```python
from build123d import *

# Parameters (mm, degrees)
ESQUISSE1_W                  = 760
ESQUISSE1_H                  = 40
BOSS_EXTRU_1_DEPTH           = 10
ENL_V_MAT_EXTRU_1_DEPTH      = 762.117599324
ENL_V_MAT_EXTRU_1_DEPTH_BACK = 762.117599324
ENL_V_MAT_EXTRU_2_DEPTH      = 762.117599324
ENL_V_MAT_EXTRU_2_DEPTH_BACK = 762.117599324
ENL_V_MAT_EXTRU_3_DEPTH      = 762.117599324
ENL_V_MAT_EXTRU_3_DEPTH_BACK = 762.117599324
ESQUISSE4_R                  = 4
CONG_1_R                     = 3
CHANFREIN1_SIZE              = 25
ENL_V_MAT_EXTRU_4_DEPTH      = 762.117599324
ENL_V_MAT_EXTRU_4_DEPTH_BACK = 762.117599324
ESQUISSE5_R                  = 2.25
ESQUISSE5_R_2                = 5
ESQUISSE5_R_3                = 2
CONG_2_R                     = 3
CONG_3_R                     = 10


with BuildPart() as part:
    # Esquisse1 → Boss.-Extru.1 (new body)
    with BuildSketch(Plane.XY):
        with Locations((380, 20)):
            Rectangle(ESQUISSE1_W, ESQUISSE1_H)
    extrude(amount=BOSS_EXTRU_1_DEPTH)

    # Esquisse2 → Enlèv. mat.-Extru.1 (cut, two sides: drawn at the far end of the back side and taken through both)
    with BuildSketch(Plane.XY.offset(10).offset(-ENL_V_MAT_EXTRU_1_DEPTH_BACK)):
        Polygon((0, 40), (60, 40), (0, 20), align=None)
    extrude(amount=ENL_V_MAT_EXTRU_1_DEPTH + ENL_V_MAT_EXTRU_1_DEPTH_BACK, mode=Mode.SUBTRACT)

    # Esquisse3 → Enlèv. mat.-Extru.2 (cut, two sides: drawn at the far end of the back side and taken through both)
    with BuildSketch(Plane.XY.offset(10).offset(-ENL_V_MAT_EXTRU_2_DEPTH_BACK)):
        with BuildLine():
            Line((75, 25), (505, 25))
            ThreePointArc((505, 25), (510, 20), (505, 15))
            Line((505, 15), (75, 15))
            ThreePointArc((75, 15), (70, 20), (75, 25))
        make_face()
    extrude(amount=ENL_V_MAT_EXTRU_2_DEPTH + ENL_V_MAT_EXTRU_2_DEPTH_BACK, mode=Mode.SUBTRACT)

    # Esquisse4 → Enlèv. mat.-Extru.3 (cut, two sides: drawn at the far end of the back side and taken through both)
    with BuildSketch(Plane.XY.offset(10).offset(-ENL_V_MAT_EXTRU_3_DEPTH_BACK)):
        with Locations(Location((530, 10, 0), (0, 0, 180))):
            Circle(ESQUISSE4_R)
        with Locations(Location((550, 30, 0), (0, 0, 180))):
            Circle(ESQUISSE4_R)
    extrude(amount=ENL_V_MAT_EXTRU_3_DEPTH + ENL_V_MAT_EXTRU_3_DEPTH_BACK, mode=Mode.SUBTRACT)

    # Congé1
    cong_1_edges = [part.edges().sort_by_distance(p)[0] for p in [
        (0, 20, 5),
        (0, 0, 5),
    ]]
    fillet(cong_1_edges, radius=CONG_1_R)

    # Chanfrein1
    chanfrein1_edges = [part.edges().sort_by_distance(p)[0] for p in [
        (760, 0, 5),
    ]]
    chamfer(chanfrein1_edges, length=CHANFREIN1_SIZE)

    # Esquisse5 → Enlèv. mat.-Extru.4 (cut, two sides: drawn at the far end of the back side and taken through both)
    with BuildSketch(Plane.XY.offset(10).offset(-ENL_V_MAT_EXTRU_4_DEPTH_BACK)):
        with Locations(Location((710, 20, 0), (0, 0, 180))):
            Circle(ESQUISSE5_R)
        with Locations(Location((668, 20, 0), (0, 0, 180))):
            Circle(ESQUISSE5_R)
        with Locations(Location((630, 30, 0), (0, 0, 180))):
            Circle(ESQUISSE5_R_2)
        with Locations(Location((605, 25, 0), (0, 0, 180))):
            Circle(ESQUISSE5_R_3)
    extrude(amount=ENL_V_MAT_EXTRU_4_DEPTH + ENL_V_MAT_EXTRU_4_DEPTH_BACK, mode=Mode.SUBTRACT)

    # Congé2
    cong_2_edges = [part.edges().sort_by_distance(p)[0] for p in [
        (760, 40, 5),
    ]]
    fillet(cong_2_edges, radius=CONG_2_R)

    # Congé3
    cong_3_edges = [part.edges().sort_by_distance(p)[0] for p in [
        (760, 25, 5),
        (735, 0, 5),
    ]]
    fillet(cong_3_edges, radius=CONG_3_R)


solid = part.part
```
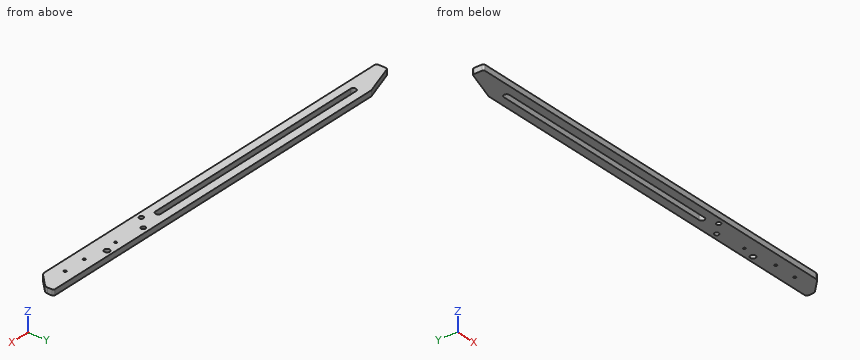
Source: CAD feature listing. Evaluate the final solid. Frame: model axes, mm. Round coordinates to 2 decimals unless told otherwise and drop trailing zeros. Order: outer loops, then holes, each group sorted by start corner. A loop starts at its lowest first (then second) coordinate and runs counter-clockwise, first axis right, second up. Notation, with made-up numbers: (78, 23.25) -> (120, 23.25) arc R23 ccw to (120, 49.25) -> close; hole circle Ø8 at (76, -38.5). An arc over 180 degrees is marked (long way). One line per item, written item: value. Start each with the question number.
Q1. Pin query (flat end, axial travel): pin 1 (1 mm diameter, centred on y = 14.5, z = 8, fed in from +X); pin 2 (5 mm diameter, centred on y = 22.5, z = 7.5, fed in from -X). Return the tip coordinate at first contact, or that it passes through.
Q2. Section query A-A (x = 111). Return the cut outline in (y, z), plus the area to 3 significant figures.
Q3. Section query B-B (z = 2). Return the cut outline in (x, y), plus the area to 3 significant figures.
Q4. Material intervals for probe 1 along Y at (x, z) = (630, 7); probe 2 along Y at (x, z) = (404.5, 4.5); probe 3 along X at (y, z) = (17, 1.75), sorted ascending.
Findings below:
1. pin 1: x = 750
1. pin 2: x = 0.92
2. outline: (0, 0) -> (15, 0) -> (15, 10) -> (0, 10) -> close; (25, 0) -> (40, 0) -> (40, 10) -> (25, 10) -> close
2. area: 300 mm²
3. outline: (0, 3) arc R3 ccw to (3, 0) -> (730.86, 0) arc R10 ccw to (737.93, 2.93) -> (757.07, 22.07) arc R10 ccw to (760, 29.14) -> (760, 37) arc R3 ccw to (757, 40) -> (60, 40) -> (2.05, 20.68) arc R3 ccw to (0, 17.84) -> close; hole (75, 15) -> (505, 15) arc R5 ccw to (505, 25) -> (75, 25) arc R5 ccw to start; hole circle Ø8 at (530, 10); hole circle Ø8 at (550, 30); hole circle Ø4 at (605, 25); hole circle Ø10 at (630, 30); hole circle Ø4.5 at (668, 20); hole circle Ø4.5 at (710, 20)
3. area: 24,900 mm²
4. probe 1: 0 to 25, 35 to 40
4. probe 2: 0 to 15, 25 to 40
4. probe 3: 0 to 71, 509 to 752
